Check sheet for the modelled part. Datum: model origin and axes. Units: mm. Round coordinates to 2 decimals unless told otherwise and drop trailing zeros. Loops run counter-clockwise (first coordinate to the right, second up) from the corner with the lowest first, then second, coordinate; pieces in that order, holes last. Notation, with made-up numbers: (19, 55.25) - (42, 55.25) arc R20 cw to (42, 70.25) - close; hole circle Ø4 at (35, -38.75). An arc over 180 degrees is marked (long way). Put each result on its own line as item: value. Start each with the question number.
```python
from build123d import *

# Parameters (mm, degrees)
PAD_DEPTH    = 1.6
SKETCH001_R  = 1.125
POCKET_DEPTH = 1.601


with BuildPart() as part:
    # Sketch → Pad (new body)
    with BuildSketch(Plane.XY):
        with BuildLine():
            Line((-20, 10), (-12, 10))
            ThreePointArc((-8, 10), (-10, 12), (-12, 10))
            Line((-8, 10), (0, 10))
            Line((0, 10), (7.5, 10))
            ThreePointArc((7.5, 10), (10, 7.5), (12.5, 10))
            Line((12.5, 10), (20, 10))
            Line((20, 10), (20, 2))
            ThreePointArc((20, -2), (22, 0), (20, 2))
            Line((20, -10), (20, -2))
            Line((20, -10), (12.5, -10))
            ThreePointArc((12.5, -10), (10, -7.5), (7.5, -10))
            Line((7.5, -10), (0, -10))
            Line((0, -10), (-8, -10))
            ThreePointArc((-12, -10), (-10, -12), (-8, -10))
            Line((-12, -10), (-20, -10))
            Line((-20, -10), (-20, -2.5))
            ThreePointArc((-20, -2.5), (-17.5, 0), (-20, 2.5))
            Line((-20, 10), (-20, 2.5))
        make_face()
    extrude(amount=PAD_DEPTH)

    # Sketch001 → Pocket (cut, through all)
    with BuildSketch(Plane.XY):
        with Locations((-10, 10)):
            Circle(SKETCH001_R)
        with Locations((-10, -10)):
            Circle(SKETCH001_R)
        with Locations((20, 0)):
            Circle(SKETCH001_R)
    extrude(amount=POCKET_DEPTH, mode=Mode.SUBTRACT)


solid = part.part
```
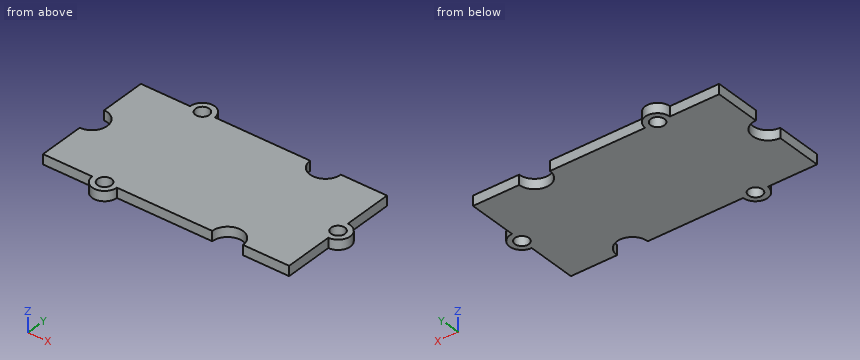
Q1. Material ranges on line 1 (Y direction, x = -10, z = 0.8) (3 decimals); line 2 (X direction, y = 0, z = 0.55) (3 decimals); line 3 (X direction, y = 6.5, z = 0.8), recorded low to high. Write a range as from..to.
Q2. Cross-section at C-C on z = 0.6. Enter the section's corners in (x, y) (3 decimals).
Q3. Depth check by flat-ended pin: pin 1 Ø0.8 at (x, z) = (1.5, 0.5) entering from +Y; pin 2 Ø0.5 at (y, z) = (4, 0.5) entering from +X; pin 3 Ø0.5 at (x, z) = (0.5, 1) entering from -Y. Enter the tip coordinate at first touch or a pass-through.
Q4. Cross-section at B-B on x = -10. Enter the section's corners in (y, z) (3 decimals).
Q5. Cross-section at A-A on y = 0. Enter the section's corners in (x, z) (3 decimals), and give its area (3 significant figures).
Q6. Cross-section at D-D on x = 10. Enter the section's corners in (y, z).
Answer list:
1. line 1: y = -12..-11.125, -8.875..8.875, 11.125..12
1. line 2: x = -17.5..18.875, 21.125..22
1. line 3: x = -20..20
2. outline: (-20, -10) - (-12, -10) arc R2 ccw to (-8, -10) - (7.5, -10) arc R2.5 cw to (12.5, -10) - (20, -10) - (20, -2) arc R2 ccw to (20, 2) - (20, 10) - (12.5, 10) arc R2.5 cw to (7.5, 10) - (-8, 10) arc R2 ccw to (-12, 10) - (-20, 10) - (-20, 2.5) arc R2.5 cw to (-20, -2.5) - close; hole circle Ø2.25 at (-10, -10); hole circle Ø2.25 at (-10, 10); hole circle Ø2.25 at (20, 0)
3. pin 1: stops at y = 10
3. pin 2: stops at x = 20
3. pin 3: stops at y = -10
4. outline: (-12, 0) - (-11.125, 0) - (-11.125, 1.6) - (-12, 1.6) - close; (-8.875, 0) - (8.875, 0) - (8.875, 1.6) - (-8.875, 1.6) - close; (11.125, 0) - (12, 0) - (12, 1.6) - (11.125, 1.6) - close
5. outline: (-17.5, 0) - (18.875, 0) - (18.875, 1.6) - (-17.5, 1.6) - close; (21.125, 0) - (22, 0) - (22, 1.6) - (21.125, 1.6) - close
5. area: 59.6 mm2
6. outline: (-7.5, 0) - (7.5, 0) - (7.5, 1.6) - (-7.5, 1.6) - close
